Design review of the part built by this model. Coordinates are the model's own, in mm. A direction names the side the tool comes from. Coordinates: 2 decimals unless noted, no trailing zeros. Write each loop counter-clockwise with the first axis right and the second up, starting at its lowest first coordinate (ties: lowest second). Pieces come first, ordered by that corner, then holes. Notation, with made-up numbers: M -21.5,41 L 34.5,41 A14 ccw 34.5,47 Z; hole C 70.25,-22.5 d10. An arc over 180 degrees is marked long. Write each question's results on one line, items separated by ' | '. Start each with the question number.
```python
from build123d import *
from build123d import SkipClean  # not in build123d's __all__

# Parameters (mm, degrees)
F0_R     = 1.15
F0_R_2   = 7.3
F0_W     = 16
F0_H     = 1.5
F0_W_2   = 6
F0_H_2   = 7.6
F1_DEPTH = 1
F3_DEPTH = 1
F4_SIZE  = 0.99999


# Not quite as in the source:
# - a fillet or chamfer is up to 0.001 mm smaller than in the source, because OpenCascade refuses the exact size


with BuildPart() as f1:
    # F0 (on Top) → F1 (new body)
    with BuildSketch(Plane.XY):
        with BuildLine():
            Line((8, -14.9), (16, -14.9))
            ThreePointArc((16, -14.9), (16.7071067812, -14.6071067812), (17, -13.9))
            Line((17, -13.9), (17, 13.9))
            ThreePointArc((17, 13.9), (16.7071067812, 14.6071067812), (16, 14.9))
            Line((16, 14.9), (3, 14.9))
            Line((3, 14.9), (-3, 14.9))
            Line((-3, 14.9), (-16, 14.9))
            ThreePointArc((-16, 14.9), (-16.7071067812, 14.6071067812), (-17, 13.9))
            Line((-17, 13.9), (-17, -13.9))
            ThreePointArc((-17, -13.9), (-16.7071067812, -14.6071067812), (-16, -14.9))
            Line((-16, -14.9), (-8, -14.9))
            Line((-8, -14.9), (8, -14.9))
        make_face()
        with BuildLine():
            Line((-8.8286237822, -10.3975032323), (-10.3326805132, -11.71576472))
            ThreePointArc((-10.3326805132, -11.71576472), (-13.1549987319, -11.5299694768), (-12.9692034887, -8.7076512581))
            Line((-12.9692034887, -8.7076512581), (-11.4651467577, -7.3893897703))
            ThreePointArc((-11.4651467577, -7.3893897703), (-8.642828539, -7.5751850136), (-8.8286237822, -10.3975032323))
        make_face(mode=Mode.SUBTRACT)
        with Locations((-11.15, 0)):
            Circle(F0_R, mode=Mode.SUBTRACT)
        with BuildLine():
            ThreePointArc((12.9692034887, -8.7076512581), (13.1549987319, -11.5299694768), (10.3326805132, -11.71576472))
            Line((10.3326805132, -11.71576472), (8.8286237822, -10.3975032323))
            ThreePointArc((8.8286237822, -10.3975032323), (8.642828539, -7.5751850136), (11.4651467577, -7.3893897703))
            Line((11.4651467577, -7.3893897703), (12.9692034887, -8.7076512581))
        make_face(mode=Mode.SUBTRACT)
        Circle(F0_R_2, mode=Mode.SUBTRACT)
        with Locations((11.15, 0)):
            Circle(F0_R, mode=Mode.SUBTRACT)
        with BuildLine():
            Line((-11.4651467577, 7.3893897703), (-12.9692034887, 8.7076512581))
            ThreePointArc((-12.9692034887, 8.7076512581), (-13.1549987319, 11.5299694768), (-10.3326805132, 11.71576472))
            Line((-10.3326805132, 11.71576472), (-8.8286237822, 10.3975032323))
            ThreePointArc((-8.8286237822, 10.3975032323), (-8.642828539, 7.5751850136), (-11.4651467577, 7.3893897703))
        make_face(mode=Mode.SUBTRACT)
        with BuildLine():
            ThreePointArc((10.3326805132, 11.71576472), (13.1549987319, 11.5299694768), (12.9692034887, 8.7076512581))
            Line((12.9692034887, 8.7076512581), (11.4651467577, 7.3893897703))
            ThreePointArc((11.4651467577, 7.3893897703), (8.642828539, 7.5751850136), (8.8286237822, 10.3975032323))
            Line((8.8286237822, 10.3975032323), (10.3326805132, 11.71576472))
        make_face(mode=Mode.SUBTRACT)
        with Locations((0, -15.65)):
            Rectangle(F0_W, F0_H)
        with Locations((0, 18.7)):
            Rectangle(F0_W_2, F0_H_2)
    extrude(amount=F1_DEPTH)

    # F2 (on face) → F3 (join)
    with BuildSketch(Plane.XY.offset(1)):
        with BuildLine():
            ThreePointArc((0, 7.3), (5.1618795027, 5.1618795027), (7.3, 0))
            ThreePointArc((7.3, 0), (5.1618795027, -5.1618795027), (0, -7.3))
            Line((0, -7.3), (0.6, -7.3))
            Line((0.6, -7.3), (0.6, -8.4787970845))
            ThreePointArc((0.6, -8.4787970845), (4.6794449698, -7.0959703195), (7.5571902637, -3.8908707661))
            ThreePointArc((7.5571902637, -3.8908707661), (7.8146834893, -3.3437586578), (8.0326290711, -2.7797248435))
            ThreePointArc((8.0326290711, -2.7797248435), (8.3823429632, -1.4093709404), (8.5, 0))
            ThreePointArc((8.5, 0), (8.3823429632, 1.4093709404), (8.0326290711, 2.7797248435))
            ThreePointArc((8.0326290711, 2.7797248435), (7.8146834893, 3.3437586578), (7.5571902637, 3.8908707661))
            ThreePointArc((7.5571902637, 3.8908707661), (4.6794449698, 7.0959703195), (0.6, 8.4787970845))
            Line((0.6, 8.4787970845), (0.6, 7.3))
            Line((0.6, 7.3), (0, 7.3))
        make_face()
        with BuildLine():
            Line((-0.6, 7.3), (0, 7.3))
            Line((0, 7.3), (0.6, 7.3))
            Line((0.6, 7.3), (0.6, 8.4787970845))
            ThreePointArc((0.6, 8.4787970845), (0, 8.5), (-0.6, 8.4787970845))
            Line((-0.6, 8.4787970845), (-0.6, 7.3))
        make_face()
        with BuildLine():
            ThreePointArc((0, -7.3), (-7.3, 0), (0, 7.3))
            Line((0, 7.3), (-0.6, 7.3))
            Line((-0.6, 7.3), (-0.6, 8.4787970845))
            ThreePointArc((-0.6, 8.4787970845), (-4.6794449698, 7.0959703195), (-7.5571902637, 3.8908707661))
            ThreePointArc((-7.5571902637, 3.8908707661), (-7.8146834893, 3.3437586578), (-8.0326290711, 2.7797248435))
            ThreePointArc((-8.0326290711, 2.7797248435), (-8.5, 0), (-8.0326290711, -2.7797248435))
            ThreePointArc((-8.0326290711, -2.7797248435), (-7.8146834893, -3.3437586578), (-7.5571902637, -3.8908707661))
            ThreePointArc((-7.5571902637, -3.8908707661), (-4.6794449698, -7.0959703195), (-0.6, -8.4787970845))
            Line((-0.6, -8.4787970845), (-0.6, -7.3))
            Line((-0.6, -7.3), (0, -7.3))
        make_face()
        with BuildLine():
            Line((0.6, -7.3), (0, -7.3))
            Line((0, -7.3), (-0.6, -7.3))
            Line((-0.6, -7.3), (-0.6, -8.4787970845))
            ThreePointArc((-0.6, -8.4787970845), (0, -8.5), (0.6, -8.4787970845))
            Line((0.6, -8.4787970845), (0.6, -7.3))
        make_face()
        with BuildLine():
            ThreePointArc((-0.6, 8.4787970845), (0, 8.5), (0.6, 8.4787970845))
            Line((0.6, 8.4787970845), (0.6, 11.4843371598))
            Line((0.6, 11.4843371598), (-0.6, 11.4843371598))
            Line((-0.6, 11.4843371598), (-0.6, 8.4787970845))
        make_face()
        with BuildLine():
            Line((0.6, -11.4843371598), (0.6, -8.4787970845))
            ThreePointArc((0.6, -8.4787970845), (0, -8.5), (-0.6, -8.4787970845))
            Line((-0.6, -8.4787970845), (-0.6, -11.4843371598))
            Line((-0.6, -11.4843371598), (0.6, -11.4843371598))
        make_face()
        with BuildLine():
            ThreePointArc((-8.0326290711, 2.7797248435), (-7.8146834893, 3.3437586578), (-7.5571902637, 3.8908707661))
            Line((-7.5571902637, 3.8908707661), (-17, 9.3426795092))
            Line((-17, 9.3426795092), (-17, 7.9570388632))
            Line((-17, 7.9570388632), (-8.0326290711, 2.7797248435))
        make_face()
        with BuildLine():
            Line((-17, -9.3426795092), (-7.5571902637, -3.8908707661))
            ThreePointArc((-7.5571902637, -3.8908707661), (-7.8146834893, -3.3437586578), (-8.0326290711, -2.7797248435))
            Line((-8.0326290711, -2.7797248435), (-17, -7.9570388632))
            Line((-17, -7.9570388632), (-17, -9.3426795092))
        make_face()
        with BuildLine():
            ThreePointArc((8.0326290711, -2.7797248435), (7.8146834893, -3.3437586578), (7.5571902637, -3.8908707661))
            Line((7.5571902637, -3.8908707661), (17, -9.3426795092))
            Line((17, -9.3426795092), (17, -7.9570388632))
            Line((17, -7.9570388632), (8.0326290711, -2.7797248435))
        make_face()
        with BuildLine():
            Line((17, 9.3426795092), (7.5571902637, 3.8908707661))
            ThreePointArc((7.5571902637, 3.8908707661), (7.8146834893, 3.3437586578), (8.0326290711, 2.7797248435))
            Line((8.0326290711, 2.7797248435), (17, 7.9570388632))
            Line((17, 7.9570388632), (17, 9.3426795092))
        make_face()
    with SkipClean():  # cleaning this boolean's faces spoils the solid; the shape is the same uncleaned
        extrude(amount=F3_DEPTH)

    # F4 (size 1 in the source; OpenCascade refuses exactly that, so slightly less here)
    f4_edges = [f1.edges().sort_by_distance(p)[0] for p in [
        (0, 11.484337, 1),
        (0, -11.484337, 1),
        (-17, -8.649859, 2),
        (17, -8.649859, 2),
        (-17, 8.649859, 2),
        (17, 8.649859, 2),
    ]]
    chamfer(f4_edges, length=F4_SIZE)


solid = f1.part
```
Item 1: We need section C-C on y = 18. State the section outline as (x, z) points, then the cut area to 3 significant figures.
Item 2: We need section D-D on z = 0.35. Count the separate pieces of the cut face and the enclosed holes in it, then the cut area to 3 significant figures.
Item 3: We need section A-A on y = -0.5. State the section outline as (x, z) points, then the cut area to 3 significant figures.
Item 4: Insertion check: pin 1 Ø4.5 at (x, y) = (-14.5, 2.5) entering from +Z; pin 2 Ø0.8 at (y, z) = (18.5, 0.5) entering from +X; pin 3 Ø11.5 at (x, y) = (0, 0) entering from -Z; pin 4 Ø0.8 at (y, z) = (18, 0.5) entering from -X. Each pin has a flat end and moves straight along its axis. Give the tip position at first contact, or say it passes through.
Item 5: For faces 4 (the flat face through (-9.591, 11.066, 0.493)), 5 (the cylindrical face through (4.73, 7.06, 1.49)), 6 (the flat face through (-0.6, -10, 1.5)), 7 (the flat face through (-12.45, -5.33, 1.49)), list the 3-axis set-ups (+Z, -Z, +X, -X, +Y, -Y) from which the entire face can be reached by the end or side of a thin tool; tool diameter is ignored.
Item 6: We need section B-B on x = 6. State the section outline as (y, z) points, then the cut area to 3 significant figures.
Item 7: Draft analysis for pull direction X (two halves, no side actions). For faces 1 (the flat face through (-12.579, 5.405, 1.493)), 2 (the flat face through (0, 22.5, 0.5)), 3 (the flat face through (-9.57, -11.047, 0.493)), state which applies: released by +X, released by -X, zero draft, split by the parting line, or undercut.
Item 8: Wall thickness on L1, parallel to Y at x = 0, z = 0.7; L2, parallel to Z at x = -4.5, y = -10; L3, parallel to X at y = 18.5, z = 0.75: over which ranges is each line inside the solid? List them lowest first.
Answer:
1) outline: M -3,0 L 3,0 L 3,1 L -3,1 Z | area: 6.00 mm^2
2) separate pieces: 1 | enclosed holes: 7 | area: 824 mm^2
3) outline: M -17,0 L -12.19,0 L -12.19,1 L -17,1 Z; M -10.11,0 L -7.28,0 L -7.28,2 L -8.49,2 L -8.49,1 L -10.11,1 Z; M 7.28,0 L 10.11,0 L 10.11,1 L 8.49,1 L 8.49,2 L 7.28,2 Z; M 12.19,0 L 17,0 L 17,1 L 12.19,1 Z | area: 17.7 mm^2
4) pin 1: stops at z = 1 | pin 2: stops at x = 3 | pin 3: passes through | pin 4: stops at x = -3
5) face 4: +Z, -Z | face 5: +Z, +Y | face 6: +Z, -Y | face 7: +Z, -X
6) outline: M -16.4,0 L -4.16,0 L -4.16,2 L -6.02,2 L -6.02,1 L -16.4,1 Z; M 4.16,0 L 14.9,0 L 14.9,1 L 6.02,1 L 6.02,2 L 4.16,2 Z | area: 26.7 mm^2
7) face 1: released by -X | face 2: zero draft | face 3: undercut
8) L1: y = -16.4 to -7.3, 7.3 to 22.5 | L2: z = 0 to 1 | L3: x = -3 to 3
